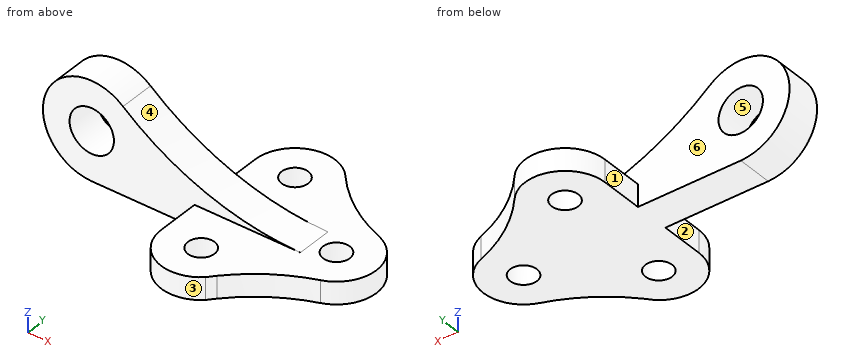
```python
from build123d import *

# Parameters (mm, degrees)
F0_R     = 6
F1_DEPTH = 10
F2_R     = 10
F3_DEPTH = 8


with BuildPart() as f1:
    # F0 (on Top) → F1 (new body)
    with BuildSketch(Plane.XY):
        with BuildLine():
            ThreePointArc((45.67737, 16.983681), (28.225108, 25.813944), (13.649464, 38.856397))
            ThreePointArc((13.649464, 38.856397), (-6.257381, 43.999525), (-18, 27.122168))
            Line((-18, 27.122168), (-18, -27.364329))
            ThreePointArc((-18, -27.364329), (-7.233419, -43.846975), (12.186406, -40.61165))
            ThreePointArc((12.186406, -40.61165), (13.552871, -38.96898), (14.965577, -37.365903))
            ThreePointArc((14.965577, -37.365903), (29.049835, -25.258696), (45.67737, -16.983681))
            ThreePointArc((45.67737, -16.983681), (57.714603, 0), (45.67737, 16.983681))
        make_face()
        with Locations((0, -27.364329)):
            Circle(F0_R, mode=Mode.SUBTRACT)
        with Locations((0, 27.122168)):
            Circle(F0_R, mode=Mode.SUBTRACT)
        with Locations((39.714603, 0)):
            Circle(F0_R, mode=Mode.SUBTRACT)
    extrude(amount=F1_DEPTH)

    # F2 (on Front) → F3 (join, symmetric)
    with BuildSketch(Plane.XZ):
        with BuildLine():
            Line((-64.32263, 0), (0, 0))
            Line((0, 0), (29.698644, 0))
            Line((29.698644, 0), (29.698644, 10))
            ThreePointArc((29.698644, 10), (-12.809858, 17.449895), (-50.251419, 38.911565))
            ThreePointArc((-50.251419, 38.911565), (-85.011449, 29.481496), (-64.32263, 0))
        make_face()
        with Locations((-64.32263, 22)):
            Circle(F2_R, mode=Mode.SUBTRACT)
    extrude(amount=F3_DEPTH, both=True)


solid = f1.part
```
Work out the finished part from the listing and answer in its coordinate system (mm). Face numbers are marked on the shaded views. A direction names the side the tool comes from. Give positions to 0.01 mm unless a question says otherwise; leave off trailing zeros. Write each loop counter-clockwise with the first axis right and the second up, starting at its lowest first coordinate (ties: lowest second). Pieces come first, ordered by that corner, then holes. Notation, with made-up numbers: (31.5, 68) - (60.5, 68) arc R21 ccw to (60.5, 85) - close; hole circle Ø6 at (-38, 54). An arc over 180 degrees is marked (long way). Use one line per item in the form item = value.
1. A cutting plane is placed at A-A (y = 0). Write down the section's boundary in (x, z), and give its area (3 significant figures).
Filled in:
outline = (-64.32, 0) - (33.71, 0) - (33.71, 10) - (29.7, 10) arc R125 cw to (-50.25, 38.91) arc R22 ccw (long way) to start; (45.71, 0) - (57.71, 0) - (57.71, 10) - (45.71, 10) - close; hole circle Ø20 at (-64.32, 22)
area = 2,730 mm^2
2. For the marked faces 1, 2 and 3, determine the directions among +Z, -Z, +X, -X, +Y, -Y from which every point of the face is accessible in a straight line to the end or side of a thin tool.
Filled in:
face_1 = +Z, -Z, -X, +Y
face_2 = +Z, -Z, -X, -Y
face_3 = +Z, -Z, -Y
3. Determine the mould class of the marked faces 4, 5 and 6 for opening direction Z: released by +Z, released by -Z, zero draft, split by the parting line, or undercut.
Filled in:
face_4 = released by +Z
face_5 = undercut
face_6 = zero draft
4. Consider L1, parallel to Y at x = 0, z = 5; L2, parallel to Z at x = -4.5, y = -37; L3, parallel to Y at x = -45, z = 3. Determine where each line is inside the solid, lowest interval first.
Filled in:
L1 = -45.36 to -33.36, -21.36 to 21.12, 33.12 to 45.12
L2 = 0 to 10
L3 = -8 to 8
5. A cutting plane is placed at B-B (z = 18). Write down the section's boundary in (x, y), and give its area (3 significant figures).
Filled in:
outline = (-85.96, -8) - (-73.49, -8) - (-73.49, 8) - (-85.96, 8) - close; (-55.16, -8) - (-14.3, -8) - (-14.3, 8) - (-55.16, 8) - close
area = 853 mm^2
6. A cutting plane is placed at D-D (z = 6). Write down the section's boundary in (x, y), and give its area (3 significant figures).
Filled in:
outline = (-79.42, -8) - (-18, -8) - (-18, -27.36) arc R18 ccw to (12.19, -40.61) arc R75 cw to (14.97, -37.37) arc R75 cw to (45.68, -16.98) arc R18 ccw to (45.68, 16.98) arc R75 cw to (13.65, 38.86) arc R18 ccw to (-18, 27.12) - (-18, 8) - (-79.42, 8) - close; hole circle Ø12 at (0, -27.36); hole circle Ø12 at (0, 27.12); hole circle Ø12 at (39.71, 0)
area = 5,270 mm^2
7. Each of these flat-tipped pins is pushed along its axis until it touches: pin 1 Ø10 at (x, y) = (4, -8) entering from +Z; pin 2 Ø3 at (y, z) = (-15, 4.5) entering from -X; pin 3 Ø22 at (x, z) = (-53, 19.5) entering from +Y. Where does it stop, or does it pass through?
Filled in:
pin_1 = 13.83
pin_2 = -18
pin_3 = 8
8. A cutting plane is placed at C-C (x = 0). Write down the section's boundary in (y, z), and give its area (3 significant figures).
Filled in:
outline = (-45.36, 0) - (-33.36, 0) - (-33.36, 10) - (-45.36, 10) - close; (-21.36, 0) - (21.12, 0) - (21.12, 10) - (8, 10) - (8, 13.58) - (-8, 13.58) - (-8, 10) - (-21.36, 10) - close; (33.12, 0) - (45.12, 0) - (45.12, 10) - (33.12, 10) - close
area = 722 mm^2
